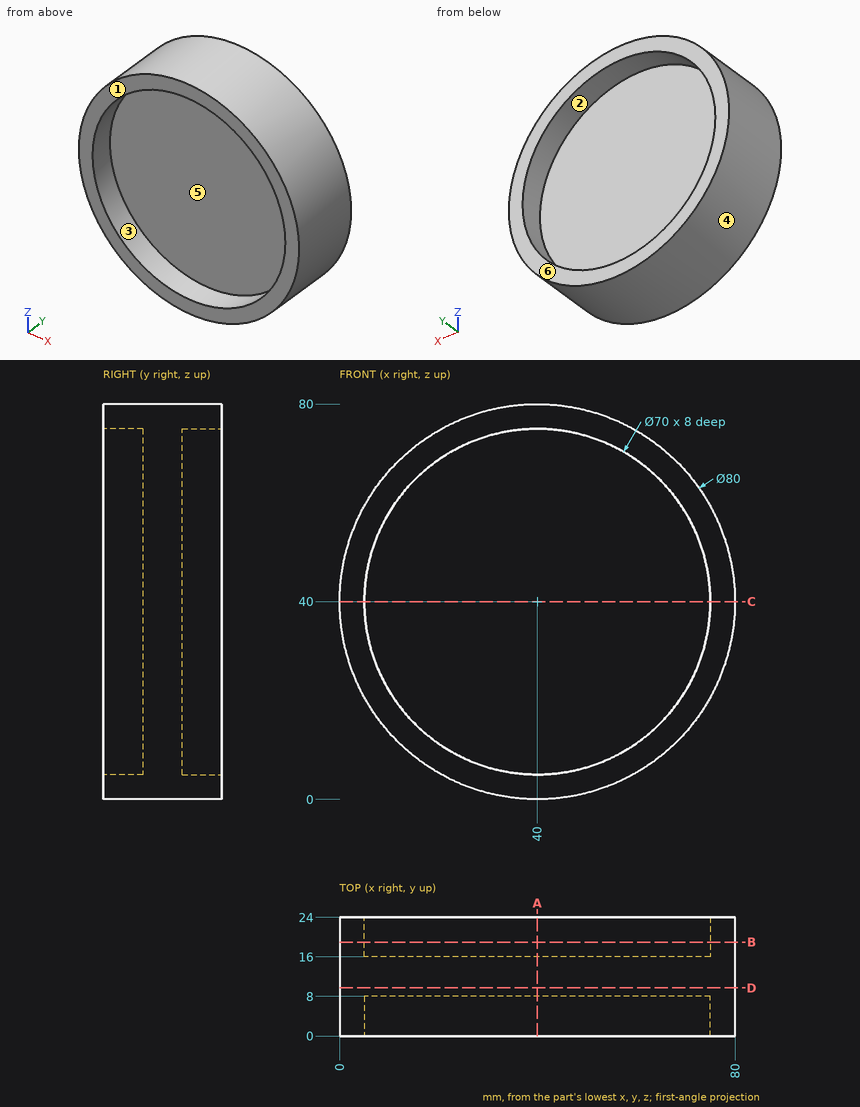
For this review, use the dimensioned drawing (mm, ordinates from the lowest corner) and the shaded views. A direction names the side the tool comes from. Round coordinates to 2 decimals unless told otherwise and drop trailing zeros. Write each loop counter-clockwise with the first axis right and the second up, starting at its lowest first coordinate (ties: lowest second). Pieces come first, ordered by that corner, then holes. Notation, with made-up numbers: (71, -2) - (127, -2) arc R30 cw to (127, 21) - close; hole circle Ø4 at (65.5, 41.5). An arc over 180 degrees is marked (long way). Use a Markdown table: item, result.
Q1. We need section C-C (z = 40). Give the boundary of the cut face in (x, y), plus the area to 3 significant figures.
Derived:
| item | result |
|---|---|
| outline | (0, 0) - (5, 0) - (5, 8) - (75, 8) - (75, 0) - (80, 0) - (80, 24) - (75, 24) - (75, 16) - (5, 16) - (5, 24) - (0, 24) - close |
| area | 800 mm2 |
Q2. Machinability: for the marked faces 1, 2 and 3, which of the approach directions +Z, -Z, +X, -X, +Y, -Y give a long, thin tool a straight path to every point of the face, cutting with its end or side? Answer none if there is none.
Derived:
| item | result |
|---|---|
| face 1 | +Z, -Z, +X, -X, -Y |
| face 2 | +Y |
| face 3 | -Y |
Q3. We need section D-D (y = 9.75). Give the boundary of the cut face in (x, z), plus the area to 3 significant figures.
Derived:
| item | result |
|---|---|
| outline | circle Ø80 at (40, 40) |
| area | 5,030 mm2 |
Q4. Wall thickness on line 1 along X through (y, z) = (20.25, 40); line 2 along Y through (x, z) = (50.5, 62.5): over which ranges is each line inside the solid? List them lowest first.
Derived:
| item | result |
|---|---|
| line 1 | x = 0 to 5, 75 to 80 |
| line 2 | y = 8 to 16 |
Q5. We need section B-B (y = 19). Give the boundary of the cut face in (x, z), plus the area to 3 significant figures.
Derived:
| item | result |
|---|---|
| outline | circle Ø80 at (40, 40); hole circle Ø70 at (40, 40) |
| area | 1,180 mm2 |
Q6. The part is to be moulded in two halves that separate along X. For the marked faces 4, 5 and 6, say which applies: pulls with the +X half, pulls with the -X half, needs draft (parallel to the pull), parting line crosses it, or undercut.
Derived:
| item | result |
|---|---|
| face 4 | parting line crosses it |
| face 5 | undercut |
| face 6 | needs draft |
Q7. We need section A-A (x = 40). Give the boundary of the cut face in (y, z), plus the area to 3 significant figures.
Derived:
| item | result |
|---|---|
| outline | (0, 0) - (24, 0) - (24, 5) - (16, 5) - (16, 75) - (24, 75) - (24, 80) - (0, 80) - (0, 75) - (8, 75) - (8, 5) - (0, 5) - close |
| area | 800 mm2 |
Q8. Clearance check with flat-ended pins moving along their axes: pin 1 (12 mm diameter, centred on y = 7.5, z = 26, fed in from -X); pin 2 (3 mm diameter, centred on x = 41.5, y = 9.5, fed in from -Z); pin 3 (1.5 mm diameter, centred on x = 49.5, y = 15, fed in from +Z). State where each tip first meets the part, or that it passes through.
Derived:
| item | result |
|---|---|
| pin 1 | stops at x = 0.81 |
| pin 2 | stops at z = 0 |
| pin 3 | stops at z = 79.03 |
